```python
from build123d import *

# Parameters (mm, degrees)
ESBO_O1_W                = 72
ESBO_O1_H                = 40
ESBO_O1_W_2              = 2.8
ESBO_O1_H_2              = 2.8
RESSALTO_EXTRUS_O1_DEPTH = 1.5


with BuildPart() as part:
    # Esboço1 → Ressalto-extrusão1 (new body)
    with BuildSketch(Plane.XY):
        Rectangle(ESBO_O1_W, ESBO_O1_H)
        with Locations((-32, 16)):
            Rectangle(ESBO_O1_W_2, ESBO_O1_H_2, mode=Mode.SUBTRACT)
        with Locations((-24, 16)):
            Rectangle(ESBO_O1_W_2, ESBO_O1_H_2, mode=Mode.SUBTRACT)
        with Locations((-24, 8)):
            Rectangle(ESBO_O1_W_2, ESBO_O1_H_2, mode=Mode.SUBTRACT)
        with Locations((32, 16)):
            Rectangle(ESBO_O1_W_2, ESBO_O1_H_2, mode=Mode.SUBTRACT)
        with Locations((-32, 8)):
            Rectangle(ESBO_O1_W_2, ESBO_O1_H_2, mode=Mode.SUBTRACT)
        with Locations((32, 8)):
            Rectangle(ESBO_O1_W_2, ESBO_O1_H_2, mode=Mode.SUBTRACT)
        with Locations((-32, 0)):
            Rectangle(ESBO_O1_W_2, ESBO_O1_H_2, mode=Mode.SUBTRACT)
        with Locations((32, 0)):
            Rectangle(ESBO_O1_W_2, ESBO_O1_H_2, mode=Mode.SUBTRACT)
        with Locations((-32, -8)):
            Rectangle(ESBO_O1_W_2, ESBO_O1_H_2, mode=Mode.SUBTRACT)
        with Locations((32, -8)):
            Rectangle(ESBO_O1_W_2, ESBO_O1_H_2, mode=Mode.SUBTRACT)
        with Locations((-32, -16)):
            Rectangle(ESBO_O1_W_2, ESBO_O1_H_2, mode=Mode.SUBTRACT)
        with Locations((32, -16)):
            Rectangle(ESBO_O1_W_2, ESBO_O1_H_2, mode=Mode.SUBTRACT)
        with Locations((-24, 0)):
            Rectangle(ESBO_O1_W_2, ESBO_O1_H_2, mode=Mode.SUBTRACT)
        with Locations((-24, -8)):
            Rectangle(ESBO_O1_W_2, ESBO_O1_H_2, mode=Mode.SUBTRACT)
        with Locations((-24, -16)):
            Rectangle(ESBO_O1_W_2, ESBO_O1_H_2, mode=Mode.SUBTRACT)
        with Locations((-16, 16)):
            Rectangle(ESBO_O1_W_2, ESBO_O1_H_2, mode=Mode.SUBTRACT)
        with Locations((-16, 8)):
            Rectangle(ESBO_O1_W_2, ESBO_O1_H_2, mode=Mode.SUBTRACT)
        with Locations((-16, 0)):
            Rectangle(ESBO_O1_W_2, ESBO_O1_H_2, mode=Mode.SUBTRACT)
        with Locations((-16, -8)):
            Rectangle(ESBO_O1_W_2, ESBO_O1_H_2, mode=Mode.SUBTRACT)
        with Locations((-16, -16)):
            Rectangle(ESBO_O1_W_2, ESBO_O1_H_2, mode=Mode.SUBTRACT)
        with Locations((-8, 16)):
            Rectangle(ESBO_O1_W_2, ESBO_O1_H_2, mode=Mode.SUBTRACT)
        with Locations((-8, 8)):
            Rectangle(ESBO_O1_W_2, ESBO_O1_H_2, mode=Mode.SUBTRACT)
        with Locations((-8, 0)):
            Rectangle(ESBO_O1_W_2, ESBO_O1_H_2, mode=Mode.SUBTRACT)
        with Locations((-8, -8)):
            Rectangle(ESBO_O1_W_2, ESBO_O1_H_2, mode=Mode.SUBTRACT)
        with Locations((-8, -16)):
            Rectangle(ESBO_O1_W_2, ESBO_O1_H_2, mode=Mode.SUBTRACT)
        with Locations((0, 16)):
            Rectangle(ESBO_O1_W_2, ESBO_O1_H_2, mode=Mode.SUBTRACT)
        with Locations((0, 8)):
            Rectangle(ESBO_O1_W_2, ESBO_O1_H_2, mode=Mode.SUBTRACT)
        Rectangle(ESBO_O1_W_2, ESBO_O1_H_2, mode=Mode.SUBTRACT)
        with Locations((0, -8)):
            Rectangle(ESBO_O1_W_2, ESBO_O1_H_2, mode=Mode.SUBTRACT)
        with Locations((0, -16)):
            Rectangle(ESBO_O1_W_2, ESBO_O1_H_2, mode=Mode.SUBTRACT)
        with Locations((8, 16)):
            Rectangle(ESBO_O1_W_2, ESBO_O1_H_2, mode=Mode.SUBTRACT)
        with Locations((8, 8)):
            Rectangle(ESBO_O1_W_2, ESBO_O1_H_2, mode=Mode.SUBTRACT)
        with Locations((8, 0)):
            Rectangle(ESBO_O1_W_2, ESBO_O1_H_2, mode=Mode.SUBTRACT)
        with Locations((8, -8)):
            Rectangle(ESBO_O1_W_2, ESBO_O1_H_2, mode=Mode.SUBTRACT)
        with Locations((8, -16)):
            Rectangle(ESBO_O1_W_2, ESBO_O1_H_2, mode=Mode.SUBTRACT)
        with Locations((16, 16)):
            Rectangle(ESBO_O1_W_2, ESBO_O1_H_2, mode=Mode.SUBTRACT)
        with Locations((16, 8)):
            Rectangle(ESBO_O1_W_2, ESBO_O1_H_2, mode=Mode.SUBTRACT)
        with Locations((16, 0)):
            Rectangle(ESBO_O1_W_2, ESBO_O1_H_2, mode=Mode.SUBTRACT)
        with Locations((16, -8)):
            Rectangle(ESBO_O1_W_2, ESBO_O1_H_2, mode=Mode.SUBTRACT)
        with Locations((16, -16)):
            Rectangle(ESBO_O1_W_2, ESBO_O1_H_2, mode=Mode.SUBTRACT)
        with Locations((24, 16)):
            Rectangle(ESBO_O1_W_2, ESBO_O1_H_2, mode=Mode.SUBTRACT)
        with Locations((24, 8)):
            Rectangle(ESBO_O1_W_2, ESBO_O1_H_2, mode=Mode.SUBTRACT)
        with Locations((24, 0)):
            Rectangle(ESBO_O1_W_2, ESBO_O1_H_2, mode=Mode.SUBTRACT)
        with Locations((24, -8)):
            Rectangle(ESBO_O1_W_2, ESBO_O1_H_2, mode=Mode.SUBTRACT)
        with Locations((24, -16)):
            Rectangle(ESBO_O1_W_2, ESBO_O1_H_2, mode=Mode.SUBTRACT)
    extrude(amount=RESSALTO_EXTRUS_O1_DEPTH)


solid = part.part
```
Read the model definition and answer for the solid it produces. Units are mm, in the model's axes. Give positions to 0.01 mm unless a question says otherwise; leave off trailing zeros. Put each result on its own line as item: value. Start each with the question number.
1. Consider line 1 along Y through (x, z) = (32, 0.35). Determine where the line is inside the solid, lowest interval first.
2. The part is cut by section A-A, the plane y = 7.5. Give the number of separate pieces and of enclosed holes in the cut face, and give its area (3 significant figures).
3. For a pull along Y with two mould halves and no side action, classify faces 1 (the flat face through (32, 6.6, 1)), 2 (the flat face through (-36, 0, 1)) as released by +Y, released by -Y, zero draft, split by the parting line, or undercut.
Final values:
1. line 1: y = -20 to -17.4, -14.6 to -9.4, -6.6 to -1.4, 1.4 to 6.6, 9.4 to 14.6, 17.4 to 20
2. separate pieces: 10
2. enclosed holes: 0
2. area: 70.2 mm²
3. face 1: undercut
3. face 2: zero draft
